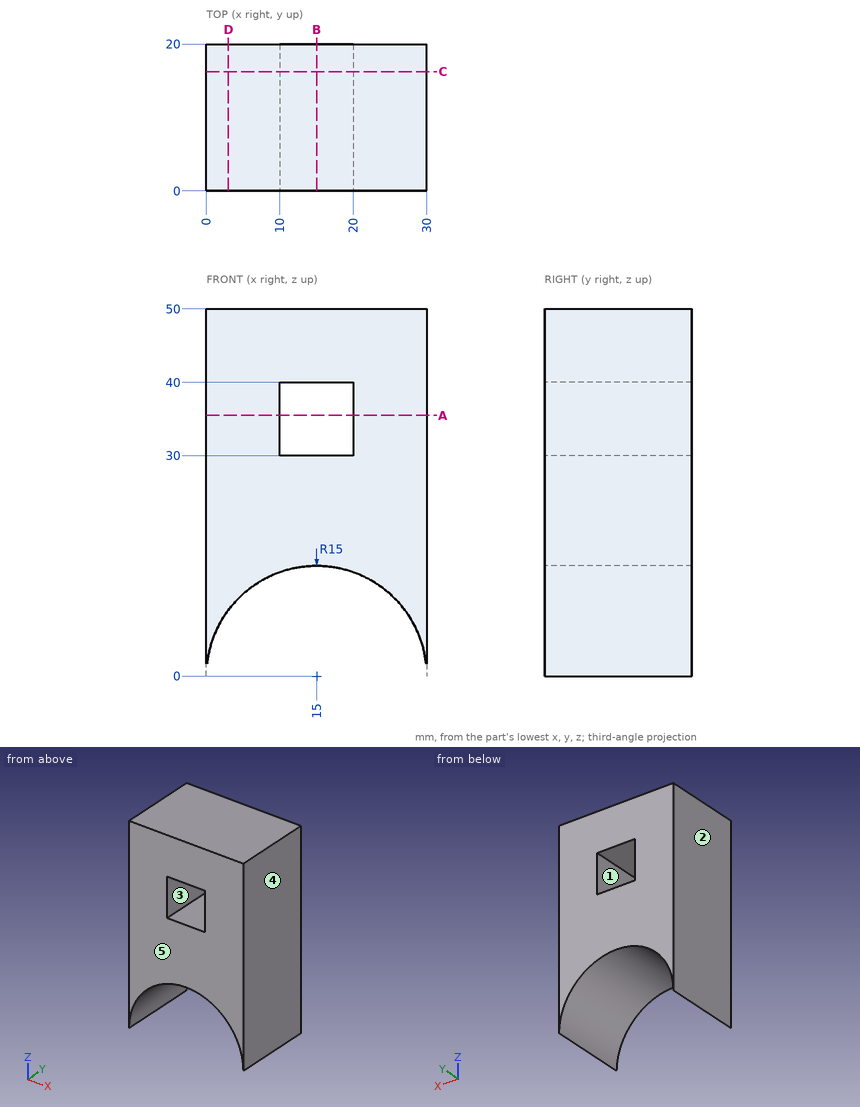
Check sheet for the drawn part. Datum: minimum x, y, z corner. Units: mm. A direction names the side the tool comes from. Round coordinates to 2 decimals unless told otherwise and drop trailing zeros. Loops run counter-clockwise (first coordinate to the right, second up) from the corner with the lowest first, then second, coordinate; pieces in that order, holes last.
Item 1: Cross-section at D-D on x = 3. Record the boundary of the cut face in (y, z).
Item 2: Gauge pin test, flat end, axial feed: pin 1 (8 mm diameter, centred on x = 15, y = 13, fed in from -Z). Record the tip position at first contact, or that the pin passes through.
Item 3: Mould release check, pull along X, two halves, no side actions. Record for the marked faces 3, 4 and 5: pulls with the +X half, pulls with the -X half, needs draft (parallel to the pull), parting line crosses it, or undercut.
Item 4: Cross-section at C-C on y = 16.25. Record the boundary of the cut face in (x, z), then the cut area to 3 significant figures.
Item 5: Cross-section at B-B on x = 15. Record the boundary of the cut face in (y, z), then the cut area to 3 significant figures.
Item 6: Thickness scan on line 1 (X direction, y = 14.25, z = 32); line 2 (Z direction, x = 16, y = 13); line 3 (Z direction, x = 17.5, y = 1.5). Record the ranges inside material, lowest first.
Item 7: Cross-section at A-A on z = 35.5. Record the boundary of the cut face in (x, y), then the cut area to 3 significant figures.
Item 8: Access from +Z, -Z, +X, -X, +Y, -Y to the whole of each face (thin tool, end or side, straight path). Record for the marked faces 1 and 2.
Answer sheet:
1. outline: (0, 9) - (20, 9) - (20, 50) - (0, 50) - close
2. pin 1: stops at z = 14.46
3. face 3: undercut
3. face 4: pulls with the +X half
3. face 5: needs draft
4. outline: (0, 0) arc R15 cw to (30, 0) - (30, 50) - (0, 50) - close; hole (10, 30) - (20, 30) - (20, 40) - (10, 40) - close
4. area: 1,050 mm2
5. outline: (0, 15) - (20, 15) - (20, 30) - (0, 30) - close; (0, 40) - (20, 40) - (20, 50) - (0, 50) - close
5. area: 500 mm2
6. line 1: x = 0 to 10, 20 to 30
6. line 2: z = 14.97 to 30, 40 to 50
6. line 3: z = 14.79 to 30, 40 to 50
7. outline: (0, 0) - (10, 0) - (10, 20) - (0, 20) - close; (20, 0) - (30, 0) - (30, 20) - (20, 20) - close
7. area: 400 mm2
8. face 1: +Y, -Y
8. face 2: +Z, -Z, -X, +Y, -Y
